```python
from build123d import *

# Parameters (mm, degrees)
SKETCH_1_R          = 2.6
EXTRUDE_1_DEPTH     = 1.5
SKETCH_2_R          = 1.1
CUT_EXTRUDE_1_DEPTH = 0.6
EXTRUDE_START       = 1
SKETCH_3_R          = 2.6
SKETCH_3_R_2        = 2.15
EXTRUDE_2_DEPTH     = 1
SKETCH_4_R          = 2.6
EXTRUDE_3_DEPTH     = 4
CUT_EXTRUDE_START   = -4.1
SKETCH_5_R          = 2.15
CUT_EXTRUDE_2_DEPTH = 4.1


with BuildPart() as part:
    # 草图1 → 凸台-拉伸1 (new body)
    with BuildSketch(Plane.XY):
        Circle(SKETCH_1_R)
    extrude(amount=EXTRUDE_1_DEPTH)

    # 草图2 → 切除-拉伸1 (cut)
    with BuildSketch(Plane(origin=(0, 0, 0), x_dir=(-1, 0, 0), z_dir=(0, 0, -1))):
        Circle(SKETCH_2_R)
    extrude(amount=-CUT_EXTRUDE_1_DEPTH, mode=Mode.SUBTRACT)

    # 草图3 → 凸台-拉伸2 (add)
    with BuildSketch(Plane(origin=(0, 0, 0), x_dir=(-1, 0, 0), z_dir=(0, 0, -1)).offset(EXTRUDE_START)):
        Circle(SKETCH_3_R)
        Circle(SKETCH_3_R_2, mode=Mode.SUBTRACT)
    extrude(amount=-EXTRUDE_2_DEPTH)

    # 草图4 → 凸台-拉伸3 (add)
    with BuildSketch(Plane.XY.offset(1.5)):
        with Locations(Location((0, 0, 0), (0, 0, 180))):
            Circle(SKETCH_4_R)
    extrude(amount=EXTRUDE_3_DEPTH)

    # 草图5 → 切除-拉伸2 (cut)
    with BuildSketch(Plane.XY.offset(5.5).offset(CUT_EXTRUDE_START)):
        with Locations(Location((0, 0, 0), (0, 0, 180))):
            Circle(SKETCH_5_R)
    extrude(amount=CUT_EXTRUDE_2_DEPTH, mode=Mode.SUBTRACT)


solid = part.part
```
Check sheet for the modelled part. Datum: model origin and axes. Units: mm. A direction names the side the tool comes from. Round coordinates to 2 decimals unless told otherwise and drop trailing zeros. Write each loop counter-clockwise with the first axis right and the second up, starting at its lowest first coordinate (ties: lowest second). Pieces come first, ordered by that corner, then holes. Notation, with made-up numbers: M 65,-26.5 L 99,-26.5 A21 cw 99,-19.5 Z; hole C 53,-32 d4. An arc over 180 degrees is marked long. Write item = value, one per line. Start each with the question number.
1. Section check C-C, the plane z = 5. Record the cut outline in (x, y).
2. Scan lines: line 1 (Y direction, x = 0, z = 4.25); line 2 (Z direction, x = 1.8, y = 0.3); line 3 (Y direction, x = -0.7, z = 1.5). Record each from-to range of solid material in increasing order. Write a range as [from, to].
3. Tool access check on faces 1 (the cylindrical face through (-1.05, 0.33, 0.3)), 2 (the flat face through (0, 0, 1.4)). Record the directions out of +Z, -Z, +X, -X, +Y, -Y that give a thin tool (end or side, any length) a straight path to the whole face; none if there is none.
4. Gauge pin test, flat ends, axial feed: pin 1 (1 mm diameter, centred on x = -0.5, y = 0, fed in from +Z); pin 2 (2.5 mm diameter, centred on x = 0, y = 0, fed in from -Z); pin 3 (1.5 mm diameter, centred on x = 1, z = 4, fed in from -Y); pin 4 (3 mm diameter, centred on y = -1, z = 2.5, fed in from +X). Record the tip position at first contact, or that the pin passes through.
5. Section check D-D, the plane z = 1.25. Record the cut outline in (x, y), then the cut area to 3 significant figures.
6. Release check for a two-part mould opening along X. For faces 3 (the cylindrical face through (2.15, -0.09, 3.42)), 4 (the flat face through (-1, 1, 0)) record: pulls with the +X half, pulls with the -X half, needs draft (parallel to the pull), parting line crosses it, or undercut.
7. Section check A-A, the plane x = 0. Record the cut outline in (y, z), then the cut area to 4 significant figures.
Results found:
q1.outline = C 0,0 d5.2; hole C 0,0 d4.3
q2.line_1 = [-2.6, -2.15], [2.15, 2.6]
q2.line_2 = [0, 1.4]
q2.line_3 = [-2.5, -2.03], [2.03, 2.5]
q3.face_1 = -Z
q3.face_2 = +Z
q4.pin_1 = 1.4
q4.pin_2 = 0
q4.pin_3 = -2.59
q4.pin_4 = 2.6
q5.outline = C 0,0 d5.2
q5.area = 21.2 mm^2
q6.face_3 = undercut
q6.face_4 = undercut
q7.outline = M -2.6,-1 L -2.15,-1 L -2.15,0 L -1.1,0 L -1.1,0.6 L 1.1,0.6 L 1.1,0 L 2.15,0 L 2.15,-1 L 2.6,-1 L 2.6,5.5 L 2.15,5.5 L 2.15,1.4 L -2.15,1.4 L -2.15,5.5 L -2.6,5.5 Z
q7.area = 10.55 mm^2
